from build123d import *

# Parameters (mm, degrees)
SKETCH1_R           = 22.300536675
BOSS_EXTRUDE1_DEPTH = 3.65
SKETCH2_R           = 2
CUT_EXTRUDE1_DEPTH  = 32.748234155


with BuildPart() as part:
    # Sketch1 → Boss-Extrude1 (new body)
    with BuildSketch(Plane(origin=(0, 0, 0), x_dir=(1, 0, 0), z_dir=(0, 1, 0))):
        with Locations(Location((0, 0, 0), (0, 0, 270))):
            Circle(SKETCH1_R)
        Polygon((-7.212489168, 0), (0, -7.212489168), (7.212489168, 0), (0, 7.212489168), align=None, mode=Mode.SUBTRACT)
    extrude(amount=BOSS_EXTRUDE1_DEPTH)

    # Sketch2 → Cut-Extrude1 (cut, through all)
    with BuildSketch(Plane(origin=(0, 3.65, 0), x_dir=(1, 0, 0), z_dir=(0, 1, 0))):
        with Locations(Location((0, 20, 0), (0, 0, 270))):
            Circle(SKETCH2_R)
        with Locations(Location((20, 0, 0), (0, 0, 270))):
            Circle(SKETCH2_R)
        with Locations(Location((0, -20, 0), (0, 0, 270))):
            Circle(SKETCH2_R)
        with Locations(Location((-20, 0, 0), (0, 0, 270))):
            Circle(SKETCH2_R)
    extrude(amount=-CUT_EXTRUDE1_DEPTH, mode=Mode.SUBTRACT)


solid = part.part
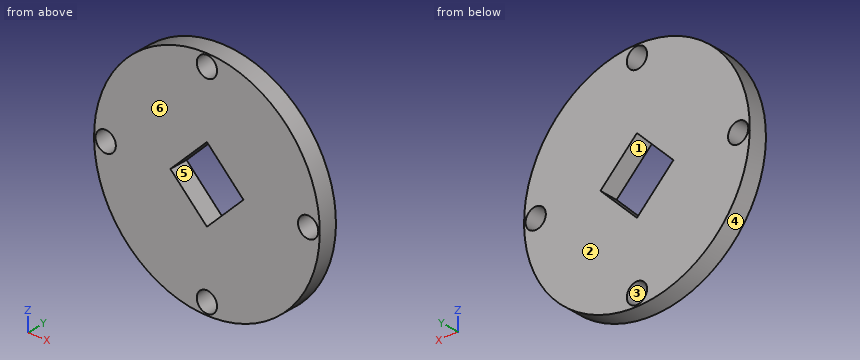
Verification items for the finished model (mm, model axes). Face numbers are marked on the shaded views. A direction names the side the tool comes from. Give positions to 0.01 mm unless a question says otherwise; leave off trailing zeros. Write each loop counter-clockwise with the first axis right and the second up, starting at its lowest first coordinate (ties: lowest second). Pieces come first, ordered by that corner, then holes. Notation, with made-up numbers: (-7.75, -1) - (49.25, -1) arc R12 ccw to (49.25, 19) - close; hole circle Ø9 at (8.25, -23). An arc over 180 degrees is marked (long way). Answer as CSV lines item,"result". Start each with the question number.
1. Sectioned sample at D-D (z = 9.5). Record the boundary of the cut face in (x, y), then the cut area to 3 significant figures.
2. Set-up check for the marked faces 5 and 6: record each of +Z, -Z, +X, -X, +Y, -Y from which the full face is reachable in a straight line by a thin tool's end or side.
3. Thickness scan on line 1 (X direction, y = 0.45, z = -1); line 2 (X direction, y = 2.8, z = -20); line 3 (X direction, y = 1.5, z = 19). Record the ranges inside material, lowest first.
4. Depth check by flat-ended pin: pin 1 (1 mm diameter, centred on y = 3, z = -15.5, fed in from +X). Enter the tip coordinate at first touch or a pass-through.
5. Sectioned sample at B-B (x = 20). Record the boundary of the cut face in (y, z).
6. Sectioned sample at A-A (y = 1.85). Record the boundary of the cut face in (x, z), then the cut area to 3 significant figures.
7. Draft check along Z on the marked faces 1, 2, 3 and 4. Enter one of: pulls with the +Z half, pulls with the -Z half, needs draft (parallel to the pull), parting line crosses it, or undercut.
8. Sectioned sample at C-C (z = -20). Record the boundary of the cut face in (x, y), then the cut area to 3 significant figures.
Derived:
1,outline,"(-20.18, 0) - (20.18, 0) - (20.18, 3.65) - (-20.18, 3.65) - close"
1,area,"147 mm²"
2,face 5,"+Y, -Y"
2,face 6,"+Z, -Z, +X, -X, -Y"
3,line 1,"-22.28 to -21.73, -18.27 to -6.21, 6.21 to 18.27, 21.73 to 22.28"
3,line 2,"-9.86 to -2, 2 to 9.86"
3,line 3,"-11.68 to -1.73, 1.73 to 11.68"
4,pin 1,"x = 16.5"
5,outline,"(0, -9.86) - (3.65, -9.86) - (3.65, -2) - (0, -2) - close; (0, 2) - (3.65, 2) - (3.65, 9.86) - (0, 9.86) - close"
6,outline,"circle Ø44.6 at (0, 0); hole circle Ø4 at (-20, 0); hole (-7.21, 0) - (0, -7.21) - (7.21, 0) - (0, 7.21) - close; hole circle Ø4 at (0, -20); hole circle Ø4 at (0, 20); hole circle Ø4 at (20, 0)"
6,area,"1,410 mm²"
7,face 1,"undercut"
7,face 2,"needs draft"
7,face 3,"undercut"
7,face 4,"parting line crosses it"
8,outline,"(-9.86, 0) - (-2, 0) - (-2, 3.65) - (-9.86, 3.65) - close; (2, 0) - (9.86, 0) - (9.86, 3.65) - (2, 3.65) - close"
8,area,"57.4 mm²"
